```python
from build123d import *

# Parameters (mm, degrees)
BOSS_EXTRUDE1_DEPTH = 90
CUT_EXTRUDE1_DEPTH  = 337
CUT_EXTRUDE3_DEPTH  = 2
CUT_EXTRUDE4_DEPTH  = 2
CUT_EXTRUDE5_DEPTH  = 2
FILLET1_R           = 5


with BuildPart() as part:
    # Sketch1 → Boss-Extrude1 (new body)
    with BuildSketch(Plane.XY):
        Polygon((-125.894137159, -28.704779811), (-125.894137159, -3.704779811), (-76.653749508, 4.977629073), (-30.691082921, 43.544885654), (69.308917079, 43.544885654), (69.308917079, 13.544885654), (154.308917079, 13.544885654), (154.308917079, -6.455114346), (61.720670681, -24.411045774), (61.720670681, -64.411045774), (31.720670681, -64.411045774), (31.720670681, -34.411045774), (-28.279329319, -34.411045774), (-28.279329319, -64.411045774), (-58.279329319, -64.411045774), (-58.279329319, -46.822112968), align=None)
    extrude(amount=-BOSS_EXTRUDE1_DEPTH)

    # Sketch2 → Cut-Extrude1 (cut)
    with BuildSketch(Plane.ZY.offset(125.894137159)):
        Polygon((-45, 119.931704065), (0, -3.704779811), (0, 165.601573034), (-28.377527092, 165.601573034), align=None)
        Polygon((-90, -3.704779811), (-45, 119.931704065), (-61.622472908, 165.601573034), (-90, 165.601573034), align=None)
    extrude(amount=-CUT_EXTRUDE1_DEPTH, mode=Mode.SUBTRACT)

    # Sketch4 → Cut-Extrude3 (cut)
    with BuildSketch(Plane(origin=(0, -0.433376912, -1.190693279), x_dir=(1, 0, 0), z_dir=(0, 0.34202014332566305, 0.9396926207859105))):
        Polygon((-60.788441179, 6.51864575), (59.308917079, 6.51864575), (59.308917079, 36.800689495), (-26.876123748, 36.800689495), align=None)
    extrude(amount=-CUT_EXTRUDE3_DEPTH, mode=Mode.SUBTRACT)

    # Sketch5 → Cut-Extrude4 (cut)
    with BuildSketch(Plane(origin=(-34.122486649, 40.665596052, 0), x_dir=(0.766044443118979, 0.6427876096865383, 0), z_dir=(-0.6427876096865383, 0.766044443118979, 0))):
        Polygon((-50.520620561, 80.535068722), (-50.520620561, 9.464931278), (-0.520620561, 21.162709123), (-0.520620561, 68.837290877), align=None)
    extrude(amount=-CUT_EXTRUDE4_DEPTH, mode=Mode.SUBTRACT)

    # Sketch7 → Cut-Extrude5 (cut)
    with BuildSketch(Plane(origin=(0, 28.492065524, -78.281306661), x_dir=(-1, 0, 0), z_dir=(0, 0.34202014332566305, -0.9396926207859105))):
        Polygon((60.788441179, -24.263167149), (26.876123748, 6.018876595), (-59.308917079, 6.018876595), (-59.308917079, -24.263167149), align=None)
    extrude(amount=-CUT_EXTRUDE5_DEPTH, mode=Mode.SUBTRACT)

    # Fillet1
    fillet1_edges = [part.edges().sort_by_distance(p)[0] for p in [
        (-125.894137159, -28.704779811, -45),
        (-125.894137159, -3.704779811, -45),
    ]]
    fillet(fillet1_edges, radius=FILLET1_R)


solid = part.part
```
Verification items for the finished model (mm, model axes). A direction names the side the tool comes from. Give positions to 0.01 mm unless a question says otherwise; leave off trailing zeros. Write each loop counter-clockwise with the first axis right and the second up, starting at its lowest first coordinate (ties: lowest second). Pieces come first, ordered by that corner, then holes. Notation, with made-up numbers: M 11.5,-1.5 L 20.5,-1.5 A12 ccw 20.5,4.5 Z; hole C 21,11 d9. An arc over 180 degrees is marked long. One line per question, with ' | ' between items.
1) Section check C-C on z = -35. Enter the section's corners in (x, y), plus the area to 3 significant figures.
Result:
outline: M -125.89,-24.87 A5 ccw -122.19,-29.7 L -58.28,-46.82 L -58.28,-64.41 L -28.28,-64.41 L -28.28,-34.41 L 31.72,-34.41 L 31.72,-64.41 L 61.72,-64.41 L 61.72,-24.41 L 154.31,-6.46 L 154.31,13.54 L 69.31,13.54 L 69.31,43.54 L -30.69,43.54 L -34.52,40.33 L -33.24,38.8 L -71.54,6.66 L -72.82,8.19 L -76.65,4.98 L -121.76,-2.98 A5 ccw -125.89,-7.9 Z | area: 16,500 mm2
2) Mould release check, pull along Y, two halves, no side actions. Record for faces 6 (the flat face through (-43, -64.411, -44)), 7 (the flat face through (-53.31, 23.28, -15.23)), 8 (the flat face through (154.309, 4, -44)), 9 (the flat face through (35.286, 4.28, -2.906)): released by +Y, released by -Y, zero draft, split by the parting line, or undercut.
Result:
face 6: released by -Y | face 7: undercut | face 8: zero draft | face 9: released by +Y
3) Section check D-D on y = 26. Enter the section's corners in (x, z).
Result:
outline: M -51.6,-79.19 L -36.59,-79.19 L -35.77,-77.06 L 59.31,-77.06 L 59.31,-79.19 L 69.31,-79.19 L 69.31,-10.81 L 59.31,-10.81 L 59.31,-12.94 L -35.77,-12.94 L -36.59,-10.81 L -51.6,-10.81 L -51.6,-15.95 L -48.49,-16.5 L -48.49,-73.5 L -51.6,-74.05 Z
4) Set-up check for faces 1 (the flat face through (-58.279, -56, -44)), 2 (the flat face through (111, 13.545, -44)), 3 (the flat face through (19, 43.545, -45)), 4 (the flat face through (-28.279, -49, -44)), 5 (the flat face through (61.721, -44, -44)): record each of +Z, -Z, +X, -X, +Y, -Y from which the full face is reachable in a straight line by a thin tool's end or side.
Result:
face 1: +Z, -Z, -X, -Y | face 2: +Z, -Z, +X, +Y | face 3: +Z, -Z, +X, -X, +Y | face 4: +Z, -Z, -Y | face 5: +Z, -Z, +X, -Y
5) Section check A-A on x = 15. Enter the section's corners in (y, z).
Result:
outline: M -34.41,-90 L -3.7,-90 L 5.69,-86.58 L 5.01,-84.7 L 33.46,-74.34 L 34.15,-76.22 L 43.54,-72.8 L 43.54,-17.2 L 34.15,-13.78 L 33.46,-15.66 L 5.01,-5.3 L 5.69,-3.42 L -3.7,0 L -34.41,0 Z
6) Gauge pin test, flat ends, axial feed: pin 1 Ø2 at (y, z) = (8.5, -18.5) entering from -X; pin 2 Ø2 at (y, z) = (23.5, -72) entering from -X; pin 3 Ø9 at (y, z) = (-51.5, -33.5) entering from -X; pin 4 Ø10 at (x, y) = (-77.5, -4) entering from +Z. Record the tip position at first contact, or that the pin passes through.
Result:
pin 1: stops at x = -73.65 | pin 2: stops at x = -52.66 | pin 3: stops at x = -58.28 | pin 4: stops at z = 0
7) Thickness scan on line 1 along X through (y, z) = (-51, -77); line 2 along Y through (x, z) = (-8, -47); line 3 along Z through (x, y) = (-30, -3). Record the ranges inside material, lowest first. Write a range as [from, to].
Result:
line 1: x = [-58.28, -28.28], [31.72, 61.72] | line 2: y = [-34.41, 43.54] | line 3: z = [-89.74, -0.26]
8) Section check B-B on y = -37. Enter the section's corners in (x, z), plus the area to 3 significant figures.
Result:
outline: M -94.94,-90 L -28.28,-90 L -28.28,0 L -94.94,0 Z; M 31.72,-90 L 61.72,-90 L 61.72,0 L 31.72,0 Z | area: 8,700 mm2
